from build123d import *

# Parameters (mm, degrees)
F0_R      = 3.175
F1_DEPTH  = 3.81
F2_R      = 3.175
F3_DEPTH  = 3.81
F4_W      = 35.3329224761
F4_H      = 3.81
F4_W_2    = 10.795
F5_DEPTH  = 38.1
F6_R      = 2.54
F7_R      = 2.54
F8_R      = 3.175
F9_DEPTH  = 3.81
F10_W     = 19.05
F10_H     = 3.81
F11_DEPTH = 38.1
F12_R     = 2.54
F13_R     = 2.54


with BuildPart() as f1:
    # F0 (on Top) → F1 (new body)
    with BuildSketch(Plane.XY):
        with BuildLine():
            ThreePointArc((25.4, -6.985), (32.385, 0), (25.4, 6.985))
            Line((25.4, 6.985), (-25.4, 6.985))
            ThreePointArc((-25.4, 6.985), (-32.385, 0), (-25.4, -6.985))
            Line((-25.4, -6.985), (25.4, -6.985))
        make_face()
        with Locations((-25.4, 0)):
            Circle(F0_R, mode=Mode.SUBTRACT)
        with Locations((25.4, 0)):
            Circle(F0_R, mode=Mode.SUBTRACT)
    extrude(amount=F1_DEPTH)

    # F2 (on face) → F3 (join)
    with BuildSketch(Plane.XY.offset(3.81)):
        with BuildLine():
            Line((-10.795, -6.985), (-10.795, 6.985))
            Line((-10.795, 6.985), (-25.4, 6.985))
            ThreePointArc((-25.4, 6.985), (-32.385, 0), (-25.4, -6.985))
            Line((-25.4, -6.985), (-10.795, -6.985))
        make_face()
        with Locations((-25.4, 0)):
            Circle(F2_R, mode=Mode.SUBTRACT)
    extrude(amount=F3_DEPTH)

    # F4 (on face) → F5 (cut)
    with BuildSketch(Plane(origin=(0, 6.985, 0), x_dir=(-1, 0, 0), z_dir=(0, 1, 0))):
        with Locations((43.066461238, 1.905)):
            Rectangle(F4_W, F4_H)
        with Locations((20.0025, 1.905)):
            Rectangle(F4_W_2, F4_H)
    extrude(amount=-F5_DEPTH, mode=Mode.SUBTRACT)

    # F6
    f6_edges = [f1.edges().sort_by_distance(p)[0] for p in [
        (-10.795, 0, 3.81),
        (-14.605, 0, 3.81),
    ]]
    fillet(f6_edges, radius=F6_R)

    # F7
    f7_edges = [f1.edges().sort_by_distance(p)[0] for p in [
        (-10.795, 0, 7.62),
        (-14.605, 0, 0),
    ]]
    fillet(f7_edges, radius=F7_R)

    # F8 (on face) → F9 (join)
    with BuildSketch(Plane.XY.offset(3.81)):
        with BuildLine():
            Line((25.4, 6.985), (10.795, 6.985))
            Line((10.795, 6.985), (10.795, -6.985))
            Line((10.795, -6.985), (25.4, -6.985))
            ThreePointArc((25.4, -6.985), (32.385, 0), (25.4, 6.985))
        make_face()
        with Locations((25.4, 0)):
            Circle(F8_R, mode=Mode.SUBTRACT)
    extrude(amount=F9_DEPTH)

    # F10 (on face) → F11 (cut)
    with BuildSketch(Plane(origin=(0, 6.985, 0), x_dir=(-1, 0, 0), z_dir=(0, 1, 0))):
        with Locations((-24.13, 1.905)):
            Rectangle(F10_W, F10_H)
    extrude(amount=-F11_DEPTH, mode=Mode.SUBTRACT)

    # F12
    f12_edges = [f1.edges().sort_by_distance(p)[0] for p in [
        (14.605, 0, 0),
        (10.795, 0, 7.62),
    ]]
    fillet(f12_edges, radius=F12_R)

    # F13
    f13_edges = [f1.edges().sort_by_distance(p)[0] for p in [
        (10.795, 0, 3.81),
        (14.605, 0, 3.81),
    ]]
    fillet(f13_edges, radius=F13_R)


solid = f1.part
Read the model definition and answer for the solid it produces. Units are mm, in the model's axes. A direction names the side the tool comes from. Give positions to 0.01 mm unless a question says otherwise; leave off trailing zeros. Loops run counter-clockwise (first coordinate to the right, second up) from the corner with the lowest first, then second, coordinate; pieces in that order, holes last. Notation, with made-up numbers: (62.25, 75) -> (77.25, 75) arc R28 cw to (77.25, 102) -> close; hole circle Ø11 at (-1, -35). An arc over 180 degrees is marked (long way). Answer as CSV lines item,"result".
Item 1: Each of these flat-tipped pins is pushed along its axis until it touches: pin 1 (3 mm diameter, centred on y = -4.5, z = 5, fed in from -X); pin 2 (7 mm diameter, centred on x = 4, y = 1, fed in from +Z); pin 3 (5 mm diameter, centred on x = 25.4, y = 0, fed in from -Z); pin 4 (2 mm diameter, centred on y = -2, z = 6, fed in from -X). Where does it stop, or does it pass through?
Returned:
pin 1,"stops at x = -31.71"
pin 2,"stops at z = 3.81"
pin 3,"passes through"
pin 4,"stops at x = -32.31"
Item 2: Find section A-A on x = 23.5. Give the vertices of the cut face in (y, z) (3 decimals), plus the area to 3 significant figures.
Returned:
outline,"(-6.985, 3.81) -> (-2.544, 3.81) -> (-2.544, 7.62) -> (-6.985, 7.62) -> close; (2.544, 3.81) -> (6.985, 3.81) -> (6.985, 7.62) -> (2.544, 7.62) -> close"
area,"33.8 mm²"
Item 3: Find section B-B on y = 0. State how many separate pieces and enclosed holes the cut face has, plus the area to 3 significant figures.
Returned:
separate pieces,"3"
enclosed holes,"0"
area,"227 mm²"
Item 4: Consider line 1 (X direction, y = 0, z = 5.95) (3 decimals); line 2 (X direction, y = 0, z = 6) (3 decimals); line 3 (Z direction, x = 29, y = -1.75). Determine where each line is inside the solid, lowest interval first. Write a range as [from, to].
Returned:
line 1,"x = [-32.385, -28.575], [-22.225, -10.787], [10.949, 22.225], [28.575, 32.385]"
line 2,"x = [-32.385, -28.575], [-22.225, -10.806], [10.967, 22.225], [28.575, 32.385]"
line 3,"z = [3.81, 7.62]"
Item 5: Determine the mould class of faces 6 (the face through (28.43, 0.95, 5.69)), 7 (the face through (32.383, -0.154, 5.688)), 8 (the face through (21, 0, 7.62)), 9 (the face through (0, -6.985, 3)) for opening direction Y: +Y half, -Y half, draft (parallel to the pull), parting line (faces both ways), or undercut.
Returned:
face 6,"undercut"
face 7,"parting line"
face 8,"draft"
face 9,"-Y half"
Item 6: Find section C-C on x = -6.5. Give the vertices of the cut face in (y, z) (3 decimals), plus the area to 3 significant figures.
Returned:
outline,"(-6.985, 0) -> (6.985, 0) -> (6.985, 3.81) -> (-6.985, 3.81) -> close"
area,"53.2 mm²"
Item 7: Find section D-D on x = -23. Give the vertices of the cut face in (y, z) (3 decimals), plus the area to 3 significant figures.
Returned:
outline,"(-6.985, 3.81) -> (-2.079, 3.81) -> (-2.079, 7.62) -> (-6.985, 7.62) -> close; (2.079, 3.81) -> (6.985, 3.81) -> (6.985, 7.62) -> (2.079, 7.62) -> close"
area,"37.4 mm²"
Item 8: For faces 1 (the face through (0, 0, 0)), 2 (the face through (21, 0, 3.81)), 3 (the face through (-21, 0, 7.62)), 4 (the face through (11.761, -0.098, 7.074)), 5 (the face through (-21, 0, 3.81)), determine the directions among +Z, -Z, +X, -X, +Y, -Y from which every point of the face is accessible in a straight line to the end or side of a thin tool.
Returned:
face 1,"-Z, +X, -X, +Y, -Y"
face 2,"-Z, +X, +Y, -Y"
face 3,"+Z, +X, -X, +Y, -Y"
face 4,"+Z, +Y, -Y"
face 5,"-Z, -X, +Y, -Y"
